from build123d import *

# Parameters (mm, degrees)
SKETCH1_R           = 4.15
SKETCH1_R_2         = 2.95
BOSS_EXTRUDE1_DEPTH = 3.6
SKETCH1_3_R         = 2.95
SKETCH1_3_R_2       = 2.47
BOSS_EXTRUDE2_DEPTH = 10.32
CHAMFER1_SIZE       = 1.75
CHAMFER1_SIZE2      = 1.318719588


with BuildPart() as part:
    # Sketch1 → Boss-Extrude1 (new body)
    with BuildSketch(Plane(origin=(0, 0, 0), x_dir=(1, 0, 0), z_dir=(0, 1, 0))):
        with Locations(Location((0, 0, 0), (0, 0, 270))):
            Circle(SKETCH1_R)
        with Locations(Location((0, 0, 0), (0, 0, 270))):
            Circle(SKETCH1_R_2, mode=Mode.SUBTRACT)
    extrude(amount=BOSS_EXTRUDE1_DEPTH)

    # Sketch1_3 → Boss-Extrude2 (add)
    with BuildSketch(Plane(origin=(0, 0, 0), x_dir=(1, 0, 0), z_dir=(0, 1, 0))):
        with Locations(Location((0, 0, 0), (0, 0, 270))):
            Circle(SKETCH1_3_R)
        with Locations(Location((0, 0, 0), (0, 0, 270))):
            Circle(SKETCH1_3_R_2, mode=Mode.SUBTRACT)
    extrude(amount=BOSS_EXTRUDE2_DEPTH)

    # Chamfer1
    chamfer1_edges = [part.edges().sort_by_distance(p)[0] for p in [
        (0, 0, -2.47),
    ]]
    chamfer1_side = [part.faces().sort_by_distance(p)[0] for p in [
        (0, 5.16, -2.47),
    ]]
    chamfer(chamfer1_edges, length=CHAMFER1_SIZE, length2=CHAMFER1_SIZE2, reference=chamfer1_side[0])


solid = part.part
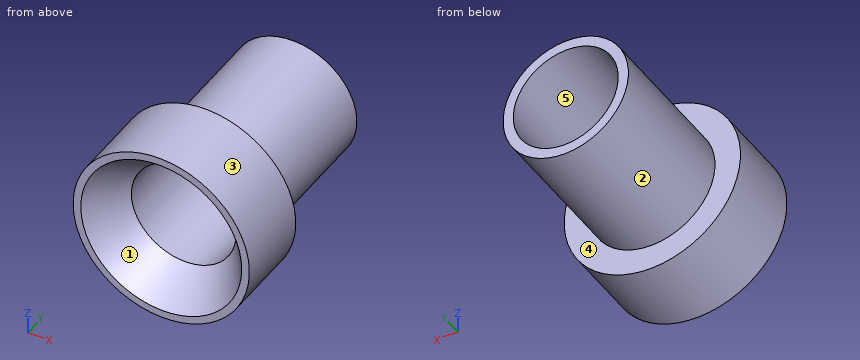
Work out the finished part from the listing and answer in its coordinate system (mm). Face numbers are marked on the shaded views. A direction names the side the tool comes from. Round coordinates to 2 decimals unless told otherwise and drop trailing zeros. Order: outer loops, then holes, each group sorted by start corner. A loop starts at its lowest first (then second) coordinate and runs counter-clockwise, first axis right, second up. Notation, with made-up numbers: M 34,73 L 67,73 A28 ccw 67,104 Z; hole C 0.5,56 d5. An arc over 180 degrees is marked long. Put each result on its own line as item: value. Start each with the question number.
Q1. A tool of negligible diameter and unlimited length cuts with its end or side. For the marked faces 1 and 2, from which of +Z, -Z, +X, -X, +Y, -Y can it reach the whole face along a straight path? Write none if from no direction.
Q2. Straight lines are drawn through the part: L1, parallel to X at y = 4.5, z = 0; L2, parallel to Z at x = -0.25, y = 3.5; L3, parallel to X at y = 2.5, z = 1.75. For each, find the intervals that lie inside material, in ascending order. Write a range as [from, to].
Q3. For a pull along X with two mould halves and no side action, classify the marked faces 3, 4 and 5 as pulls with the +X half, pulls with the -X half, needs draft (parallel to the pull), parting line crosses it, or undercut.
Q4. Section A-A, the plane x = 0 is taken. Write down the section's boundary in (y, z).
Q5. Section C-C, the plane y = 7.75 is taken. Write down the section's boundary in (x, z).
Q6. Section D-D, the plane y = 3 is taken. Write down the section's boundary in (x, z).
Q7. Section B-B, the plane z = 0 is taken. Write down the section's boundary in (x, y).
Q8. Flat-ended cylindrical pins translate along their axes: pin 1 (4 mm diameter, centred on y = 6, z = 1, fed in from +X); pin 2 (3 mm diameter, centred on y = 5, z = 1.5, fed in from +X); pin 3 (1.5 mm diameter, centred on x = -1.5, z = 0, fed in from -Y); pin 4 (4 mm diameter, centred on x = 2, y = 8, fed in from +Z). Find the tip coordinate at first contact, or state that the pin passes through.
Findings below:
1. face 1: -Y
1. face 2: +Y
2. L1: x = [-2.95, -2.47], [2.47, 2.95]
2. L2: z = [-4.14, -2.46], [2.46, 4.14]
2. L3: x = [-3.76, -1.74], [1.74, 3.76]
3. face 3: parting line crosses it
3. face 4: needs draft
3. face 5: undercut
4. outline: M 0,-4.15 L 3.6,-4.15 L 3.6,-2.95 L 10.32,-2.95 L 10.32,-2.47 L 1.75,-2.47 L 0,-3.79 Z; M 0,3.79 L 1.75,2.47 L 10.32,2.47 L 10.32,2.95 L 3.6,2.95 L 3.6,4.15 L 0,4.15 Z
5. outline: C 0,0 d5.9; hole C 0,0 d4.94
6. outline: C 0,0 d8.3; hole C 0,0 d4.94
7. outline: M -4.15,0 L -3.79,0 L -2.47,1.75 L -2.47,10.32 L -2.95,10.32 L -2.95,3.6 L -4.15,3.6 Z; M 2.47,1.75 L 3.79,0 L 4.15,0 L 4.15,3.6 L 2.95,3.6 L 2.95,10.32 L 2.47,10.32 Z
8. pin 1: stops at x = 2.95
8. pin 2: stops at x = 4.04
8. pin 3: passes through
8. pin 4: stops at z = 2.95
